```python
from build123d import *

# Parameters (mm, degrees)
SKETCH1_R            = 7.6
BOSS_EXTRUDE1_DEPTH  = 25
SKETCH2_W            = 30
SKETCH2_H            = 27
BOSS_EXTRUDE2_DEPTH  = 25
SKETCH3_R            = 7.6
BOSS_EXTRUDE3_DEPTH  = 2
CHAMFER1_SIZE        = 5
SKETCH5_W            = 25
SKETCH5_H            = 4
BOSS_EXTRUDE4_DEPTH  = 15
SKETCH6_R            = 2.25
CUT_EXTRUDE2_DEPTH   = 15
FILLET1_R            = 10
FILLET1_OF_MIRROR2_R = 10
SKETCH7_R            = 2.25
CUT_EXTRUDE3_DEPTH   = 15
CUT_EXTRUDE4_DEPTH   = 15


with BuildPart() as part:
    # Sketch1 → Boss-Extrude1 (new body)
    with BuildSketch(Plane.XY):
        with BuildLine():
            Line((-90, 0), (-90, 17))
            Line((-90, 17), (90, 17))
            Line((90, 17), (90, 0))
            ThreePointArc((90, 0), (80, -10), (70, 0))
            Line((70, 0), (70, 13))
            Line((70, 13), (-70, 13))
            Line((-70, 13), (-70, 0))
            ThreePointArc((-70, 0), (-80, -10), (-90, 0))
        make_face()
        with Locations((-80, 0)):
            Circle(SKETCH1_R, mode=Mode.SUBTRACT)
        with Locations((80, 0)):
            Circle(SKETCH1_R, mode=Mode.SUBTRACT)
    extrude(amount=BOSS_EXTRUDE1_DEPTH)

    # Sketch2 → Boss-Extrude2 (add)
    with BuildSketch(Plane(origin=(0, 0, 0), x_dir=(-1, 0, 0), z_dir=(0, 0, -1))):
        with Locations((-31, 3.5)):
            Rectangle(SKETCH2_W, SKETCH2_H)
    extrude(amount=-BOSS_EXTRUDE2_DEPTH)

    # Sketch3 → Boss-Extrude3 (add)
    with BuildSketch(Plane(origin=(0, 0, 0), x_dir=(-1, 0, 0), z_dir=(0, 0, -1))):
        with BuildLine():
            Line((80, -10), (-12, -10))
            Line((-12, -10), (-42, -10))
            Line((-42, -10), (-80, -10))
            ThreePointArc((-80, -10), (-87.071067812, -7.071067812), (-90, 0))
            Line((-90, 0), (-90, 17))
            Line((-90, 17), (90, 17))
            Line((90, 17), (90, 0))
            ThreePointArc((90, 0), (87.071067812, -7.071067812), (80, -10))
        make_face()
        with Locations((80, 0)):
            Circle(SKETCH3_R, mode=Mode.SUBTRACT)
        with Locations((-80, 0)):
            Circle(SKETCH3_R, mode=Mode.SUBTRACT)
    boss_extrude3 = extrude(amount=-BOSS_EXTRUDE3_DEPTH)

    # Mirror1: Boss-Extrude3 across plane
    add(boss_extrude3.mirror(Plane.XY.offset(12.5)))

    # Chamfer1
    chamfer1_edges = [part.edges().sort_by_distance(p)[0] for p in [
        (70, 13, 12.5),
        (-70, 13, 12.5),
    ]]
    chamfer(chamfer1_edges, length=CHAMFER1_SIZE)

    # Sketch5 → Boss-Extrude4 (add)
    with BuildSketch(Plane.ZY.offset(90)):
        with Locations((12.5, 15)):
            Rectangle(SKETCH5_W, SKETCH5_H)
    boss_extrude4 = extrude(amount=BOSS_EXTRUDE4_DEPTH)

    # Sketch6 → Cut-Extrude2 (cut)
    with BuildSketch(Plane(origin=(0, 13, 0), x_dir=(-1, 0, 0), z_dir=(0, -1, 0))):
        with Locations((97.5, -12.5)):
            Circle(SKETCH6_R)
    cut_extrude2 = extrude(amount=-CUT_EXTRUDE2_DEPTH, mode=Mode.SUBTRACT)

    # Fillet1
    fillet1_edges = [part.edges().sort_by_distance(p)[0] for p in [
        (-105, 15, 0),
        (-105, 15, 25),
    ]]
    fillet(fillet1_edges, radius=FILLET1_R)

    # Mirror2: Boss-Extrude4 across plane
    add(boss_extrude4.mirror(Plane(origin=(0, 0, 0), x_dir=(0, 0, 1), z_dir=(1, 0, 0))))

    # Fillet1 of Mirror2
    fillet1_of_mirror2_edges = [part.edges().sort_by_distance(p)[0] for p in [
        (105, 15, 0),
        (105, 15, 25),
    ]]
    fillet(fillet1_of_mirror2_edges, radius=FILLET1_OF_MIRROR2_R)

    # Mirror4: Cut-Extrude2 across plane
    add(cut_extrude2.mirror(Plane(origin=(0, 0, 0), x_dir=(0, 0, 1), z_dir=(1, 0, 0))), mode=Mode.SUBTRACT)

    # Sketch7 → Cut-Extrude3 (cut)
    with BuildSketch(Plane(origin=(0, 17, 0), x_dir=(1, 0, 0), z_dir=(0, 1, 0))):
        with Locations((-57.5, -12.5)):
            Circle(SKETCH7_R)
        with Locations((57.5, -12.5)):
            Circle(SKETCH7_R)
    extrude(amount=-CUT_EXTRUDE3_DEPTH, mode=Mode.SUBTRACT)

    # Sketch8 → Cut-Extrude4 (cut)
    with BuildSketch(Plane.XZ.offset(10)):
        with BuildLine():
            Line((21.95, 19), (20, 19))
            Line((20, 19), (20, 17.05))
            ThreePointArc((20, 17.05), (21.378858223, 17.621141777), (21.95, 19))
        make_face()
        with BuildLine():
            Line((20, 17.05), (20, 19))
            Line((20, 19), (21.95, 19))
            ThreePointArc((21.95, 19), (18.621141777, 20.378858223), (20, 17.05))
        make_face()
        with BuildLine():
            ThreePointArc((43.95, 19), (42, 20.95), (40.05, 19))
            Line((40.05, 19), (42, 19))
            Line((42, 19), (42, 17.05))
            ThreePointArc((42, 17.05), (43.378858223, 17.621141777), (43.95, 19))
        make_face()
        with BuildLine():
            Line((42, 19), (40.05, 19))
            ThreePointArc((40.05, 19), (40.621141777, 17.621141777), (42, 17.05))
            Line((42, 17.05), (42, 19))
        make_face()
        with BuildLine():
            ThreePointArc((42, 7.95), (40.621141777, 7.378858223), (40.05, 6))
            Line((40.05, 6), (42, 6))
            Line((42, 6), (42, 7.95))
        make_face()
        with BuildLine():
            Line((42, 6), (40.05, 6))
            ThreePointArc((40.05, 6), (42, 4.05), (43.95, 6))
            ThreePointArc((43.95, 6), (43.378858223, 7.378858223), (42, 7.95))
            Line((42, 7.95), (42, 6))
        make_face()
        with BuildLine():
            ThreePointArc((21.95, 6), (21.378858223, 7.378858223), (20, 7.95))
            Line((20, 7.95), (20, 6))
            Line((20, 6), (21.95, 6))
        make_face()
        with BuildLine():
            Line((20, 6), (20, 7.95))
            ThreePointArc((20, 7.95), (18.621141777, 4.621141777), (21.95, 6))
            Line((21.95, 6), (20, 6))
        make_face()
    extrude(amount=-CUT_EXTRUDE4_DEPTH, mode=Mode.SUBTRACT)


solid = part.part
```
The model under review builds one solid part; all positions refer to its coordinate system, in mm. A direction names the side the tool comes from. Give positions to 0.01 mm unless a question says otherwise; leave off trailing zeros. Write each loop counter-clockwise with the first axis right and the second up, starting at its lowest first coordinate (ties: lowest second). Pieces come first, ordered by that corner, then holes. Notation, with made-up numbers: (-38, -21) -> (-26, -21) arc R31 ccw to (-26, 4) -> close; hole circle Ø2 at (83, 33). An arc over 180 degrees is marked (long way). Answer in a Markdown table with one row per item.
1) For L1, parallel to X at y = 15.5, z = 12.5; L2, parallel to X at y = 7.75, z = 22.75; L3, parallel to X at y = -8.25, z = 9.5, list the stretches that pass through material, from the lowest coordinate up. Write a range as [from, to].
Worked answers:
| item | result |
|---|---|
| L1 | [-105, -99.75], [-95.25, -59.75], [-55.25, 55.25], [59.75, 95.25], [99.75, 105] |
| L2 | [-90, -70], [16, 46], [70, 90] |
| L3 | [-85.65, -74.35], [16, 46], [74.35, 85.65] |
2) Add section B-B on x = -57.5. State the section outline as (y, z) points, plus the area to 3 significant figures.
Worked answers:
| item | result |
|---|---|
| outline | (-10, 0) -> (17, 0) -> (17, 10.25) -> (13, 10.25) -> (13, 2) -> (-10, 2) -> close; (-10, 23) -> (13, 23) -> (13, 14.75) -> (17, 14.75) -> (17, 25) -> (-10, 25) -> close |
| area | 174 mm² |
3) Add section D-D on x = 13. State the section outline as (y, z) points, plus the area to 3 significant figures.
Worked answers:
| item | result |
|---|---|
| outline | (-10, 0) -> (17, 0) -> (17, 25) -> (-10, 25) -> (-10, 23) -> (13, 23) -> (13, 2) -> (-10, 2) -> close |
| area | 192 mm² |
4) Mouldability with a two-part tool opening along X and no side actions: class faces 4 (the flat face through (-33, 2, 23)), 5 (the cylindrical face through (101.99, 15.03, 22.15)), 6 (the flat face through (94, 13, 12)) as +X half, -X half, draft (parallel to the pull), parting line (faces both ways), or undercut.
Worked answers:
| item | result |
|---|---|
| face 4 | undercut |
| face 5 | +X half |
| face 6 | draft |
5) Add section A-A on y = 3. Count the separate pieces of the cut face and the enclosed holes in it, plus the area to 3 significant figures.
Worked answers:
| item | result |
|---|---|
| separate pieces | 3 |
| enclosed holes | 6 |
| area | 1,440 mm² |
6) Clearance check with flat-ended pins moving along their axes: P1, Ø6, axis at x = -57.5, z = 12.5, coming from the -Y side; P2, Ø6.5, axis at y = 4, z = 6.5, coming from the +X side; P3, Ø14.5, axis at y = 4, z = 6.5, coming from the -X side; P4, Ø3.5, axis at x = 57.5, z = 12.5, coming from the +Y side. State where each tip first meets the part, or that it passes through.
Worked answers:
| item | result |
|---|---|
| P1 | y = 13 |
| P2 | x = 90 |
| P3 | x = -90 |
| P4 | through |
7) Tool access review of faces 1 (the cylindrical face through (-80, -10, 12)), 2 (the flat face through (-90, 6, 12)), 3 (the cylindrical face through (-59.748, 15.028, 12.401)): name each direction out of +Z, -Z, +X, -X, +Y, -Y from which nothing blocks a thin tool from reaching the whole face with its end or side.
Worked answers:
| item | result |
|---|---|
| face 1 | -Y |
| face 2 | +Z, -Z, -X, -Y |
| face 3 | +Y, -Y |
